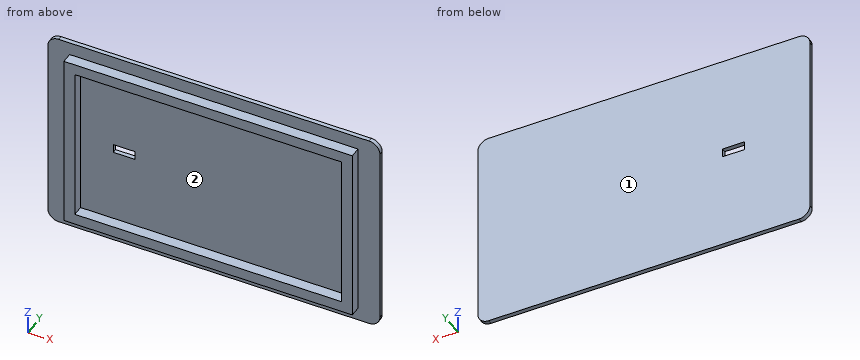
from build123d import *

# Parameters (mm, degrees)
SKETCH1_W           = 76
SKETCH1_H           = 47
BOSS_EXTRUDE1_DEPTH = 1
SKETCH2_W           = 66
SKETCH2_H           = 41
SKETCH2_W_2         = 61
SKETCH2_H_2         = 36
BOSS_EXTRUDE2_DEPTH = 2.5
FILLET1_R           = 2.5
SKETCH4_W           = 5
SKETCH4_H           = 2
CUT_EXTRUDE1_DEPTH  = 1


with BuildPart() as part:
    # Sketch1 → Boss-Extrude1 (new body)
    with BuildSketch(Plane(origin=(0, 0, 0), x_dir=(1, 0, 0), z_dir=(0, 1, 0))):
        Rectangle(SKETCH1_W, SKETCH1_H)
    extrude(amount=-BOSS_EXTRUDE1_DEPTH)

    # Sketch2 → Boss-Extrude2 (add)
    with BuildSketch(Plane.XZ.offset(1)):
        Rectangle(SKETCH2_W, SKETCH2_H)
        Rectangle(SKETCH2_W_2, SKETCH2_H_2, mode=Mode.SUBTRACT)
    extrude(amount=BOSS_EXTRUDE2_DEPTH)

    # Fillet1
    fillet1_edges = [part.edges().sort_by_distance(p)[0] for p in [
        (38, -0.5, 23.5),
        (-38, -0.5, 23.5),
        (-38, -0.5, -23.5),
        (38, -0.5, -23.5),
    ]]
    fillet(fillet1_edges, radius=FILLET1_R)

    # Sketch4 → Cut-Extrude1 (cut)
    with BuildSketch(Plane(origin=(0, 0, 0), x_dir=(1, 0, 0), z_dir=(0, 1, 0))):
        with Locations((-20.5, 0)):
            Rectangle(SKETCH4_W, SKETCH4_H)
    extrude(amount=-CUT_EXTRUDE1_DEPTH, mode=Mode.SUBTRACT)


solid = part.part
CAD build for the part. Positions are in the model's coordinates, mm. Face numbers are marked on the shaded views. Round coordinates to 2 decimals unless told otherwise and drop trailing zeros. Write each loop counter-clockwise with the first axis right and the second up, starting at its lowest first coordinate (ties: lowest second). Pieces come first, ordered by that corner, then holes.
(1) Probe line 1 along X through (y, z) = (-2.85, -16); line 2 along X through (y, z) = (-0.4, 0); line 3 along Z through (x, y) = (11, -2.7). List the from-to ranges inside material, lowest first.
(2) Drop flat-ended pins along their axis: P1, Ø2, axis at x = 4, y = -1.5, coming from the +Z side; P2, Ø1.2, axis at y = -2, z = -5, coming from the +X side; P3, Ø2, axis at y = -3, z = 7, coming from the -X side; P4, Ø2, axis at x = -20, y = -2.5, coming from the -Z side. Give the stop position or say it passes through.
(3) Slice it at A-A, the plane y = -2.4. Write the cut outline in (x, z), and give its area (3 significant figures).
(4) Slice it at B-B, the plane z = -15. Write the cut outline in (x, y), and give its area (3 significant figures).
(5) Slice it at C-C, the plane x = -29.5. Write the cut outline in (y, z), and give its area (3 significant figures).
(6) Mould opens along Z. For the marked faces 1 and 2 say: pulls with the +Z half, pulls with the -Z half, needs draft (parallel to the pull), parting line crosses it, or undercut.
From the geometry:
1. line 1: x = -33 to -30.5, 30.5 to 33
1. line 2: x = -38 to -23, -18 to 38
1. line 3: z = -20.5 to -18, 18 to 20.5
2. P1: stops at z = 23.5
2. P2: stops at x = 33
2. P3: stops at x = -33
2. P4: stops at z = -20.5
3. outline: (-33, -20.5) - (33, -20.5) - (33, 20.5) - (-33, 20.5) - close; hole (-30.5, -18) - (30.5, -18) - (30.5, 18) - (-30.5, 18) - close
3. area: 510 mm2
4. outline: (-38, -1) - (-33, -1) - (-33, -3.5) - (-30.5, -3.5) - (-30.5, -1) - (30.5, -1) - (30.5, -3.5) - (33, -3.5) - (33, -1) - (38, -1) - (38, 0) - (-38, 0) - close
4. area: 88.5 mm2
5. outline: (-3.5, -20.5) - (-1, -20.5) - (-1, -23.5) - (0, -23.5) - (0, 23.5) - (-1, 23.5) - (-1, 20.5) - (-3.5, 20.5) - (-3.5, 18) - (-1, 18) - (-1, -18) - (-3.5, -18) - close
5. area: 59.5 mm2
6. face 1: needs draft
6. face 2: undercut
